For this review, use the dimensioned drawing (mm, ordinates from the lowest corner) and the shaded views. A direction names the side the tool comes from. Coordinates: 2 decimals unless noted, no trailing zeros. Write each loop counter-clockwise with the first axis right and the second up, starting at its lowest first coordinate (ties: lowest second). Pieces come first, ordered by that corner, then holes. Notation, with made-up numbers: (-26.75, 0.25) - (8.25, 0.25) arc R17 ccw to (8.25, 19.25) - close; hole circle Ø10 at (76, 61). An arc over 180 degrees is marked (long way). Use one line per item in the form item = value. Start each with the question number.
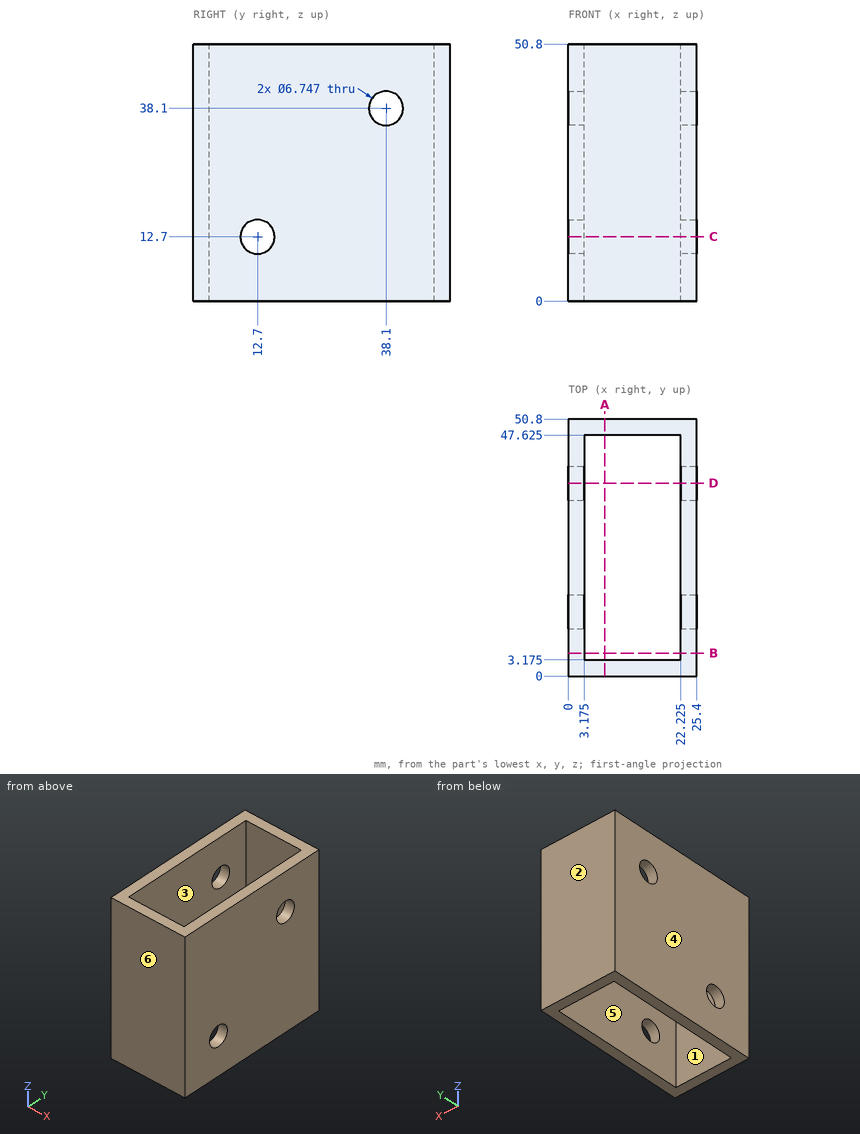
1. Take a section at D-D (y = 38.1). State the section outline as (x, z) points (1 decimal).
2. For L1, parallel to Y at x = 9.5, z = 48.5 (3 decimals); L2, parallel to X at y = 13.5, z = 33 (3 decimals); L3, parallel to Y at x = 1.55, z = 38.1, list the stretches that pass through material, from the lowest coordinate up.
3. For P1, Ø4, axis at y = 38.1, z = 38.1, coming from the -X side, flat-tipped, find the tip position at first contact; note if it passes through.
4. Take a section at C-C (z = 12.7). State the section outline as (x, y) points (1 decimal), plus the area to 3 significant figures.
5. Take a section at B-B (y = 4.5). State the section outline as (x, z) points (3 decimals).
6. The part is to be moulded in two halves that separate along X. For the marked faces 1, 2, 3 and 4, say which applies: released by +X, released by -X, zero draft, split by the parting line, or undercut.
7. Take a section at A-A (x = 7.25). State the section outline as (y, z) points (3 decimals).
8. For the marked faces 5 and 6, list the 3-axis set-ups (+Z, -Z, +X, -X, +Y, -Y) from which the entire face can be reached by the end or side of a thin tool; tool diameter is ignored.
Returned:
q1.outline = (0, 0) - (3.2, 0) - (3.2, 34.7) - (0, 34.7) - close; (0, 41.5) - (3.2, 41.5) - (3.2, 50.8) - (0, 50.8) - close; (22.2, 0) - (25.4, 0) - (25.4, 34.7) - (22.2, 34.7) - close; (22.2, 41.5) - (25.4, 41.5) - (25.4, 50.8) - (22.2, 50.8) - close
q2.L1 = 0 to 3.175, 47.625 to 50.8
q2.L2 = 0 to 3.175, 22.225 to 25.4
q2.L3 = 0 to 34.73, 41.47 to 50.8
q3.P1 = through
q4.outline = (0, 0) - (25.4, 0) - (25.4, 9.3) - (22.2, 9.3) - (22.2, 3.2) - (3.2, 3.2) - (3.2, 9.3) - (0, 9.3) - close; (0, 16.1) - (3.2, 16.1) - (3.2, 47.6) - (22.2, 47.6) - (22.2, 16.1) - (25.4, 16.1) - (25.4, 50.8) - (0, 50.8) - close
q4.area = 401 mm²
q5.outline = (0, 0) - (3.175, 0) - (3.175, 50.8) - (0, 50.8) - close; (22.225, 0) - (25.4, 0) - (25.4, 50.8) - (22.225, 50.8) - close
q6.face_1 = undercut
q6.face_2 = zero draft
q6.face_3 = undercut
q6.face_4 = released by -X
q7.outline = (0, 0) - (3.175, 0) - (3.175, 50.8) - (0, 50.8) - close; (47.625, 0) - (50.8, 0) - (50.8, 50.8) - (47.625, 50.8) - close
q8.face_5 = +Z, -Z
q8.face_6 = +Z, -Z, +X, -X, -Y
